Input: part model. Units: mm. Frame: model coordinates. Coordinates: 2 decimals unless noted, no trailing zeros. Write each loop counter-clockwise with the first axis right and the second up, starting at its lowest first coordinate (ties: lowest second). Pieces come first, ordered by that corner, then holes. Notation, with made-up numbers: (1.5, -36.5) - (24.5, -36.5) arc R28 ccw to (24.5, -13.5) - close; hole circle Ø9 at (-3.5, 89.25). An arc over 180 degrees is marked (long way). One line per question, with ' | ' between items. Start each with the question number.
1) Section query C-C on z = -72.5. Return loops of the section in (x, y).
2) Section query D-D on y = 1.4. Give the number of separate pieces and of enclosed holes in the cut face, and give its area (3 significant figures).
3) Line query: line 1 (X direction, y = 1.5, z = -33.5); line 2 (X direction, y = 0.4, z = 25); line 3 (X direction, y = 1.3, z = 7). Output: solid intervals per line, ascending.
4) Section query A-A on z = -9. Return loops of the section in (x, y).
5) First-contact query: P1, Ø1.5, axis at x = 33, z = 14.5, coming from the -Y side. Flat tip, straight axial feed; report the tip coordinate or a pass-through.
6) Section query B-B on x = 53. Return loops of the section in (y, z), and give its area (3 significant figures).
```python
from build123d import *

# Parameters (mm, degrees)
SKETCH3_W           = 200
SKETCH3_H           = 200
BOSS_EXTRUDE1_DEPTH = 3
SKETCH4_R           = 1.5
SKETCH4_R_2         = 23.5
SKETCH4_R_3         = 60
SKETCH4_W           = 30
SKETCH4_H           = 70
CUT_EXTRUDE1_DEPTH  = 5
FILLET1_R           = 5
FILLET2_R           = 2
CUT_EXTRUDE2_START  = -1
CUT_EXTRUDE2_DEPTH  = 1


with BuildPart() as part:
    # Sketch3 → Boss-Extrude1 (new body)
    with BuildSketch(Plane(origin=(0, 0, 0), x_dir=(1, 0, 0), z_dir=(0, 1, 0))):
        Rectangle(SKETCH3_W, SKETCH3_H)
    extrude(amount=BOSS_EXTRUDE1_DEPTH)

    # Sketch4 → Cut-Extrude1 (cut)
    with BuildSketch(Plane(origin=(0, 3, 0), x_dir=(1, 0, 0), z_dir=(0, 1, 0))):
        with Locations(Location((92, 92, 0), (0, 0, 270))):
            Circle(SKETCH4_R)
        with Locations(Location((92, -92, 0), (0, 0, 270))):
            Circle(SKETCH4_R)
        with Locations(Location((-92, -92, 0), (0, 0, 270))):
            Circle(SKETCH4_R)
        with Locations(Location((-92, 92, 0), (0, 0, 270))):
            Circle(SKETCH4_R)
        with Locations(Location((92, -25, 0), (0, 0, 270))):
            Circle(SKETCH4_R)
        with Locations(Location((93.5, -65, 0), (0, 0, 270))):
            Circle(SKETCH4_R)
        with Locations(Location((17, -93, 0), (0, 0, 270))):
            Circle(SKETCH4_R)
        with Locations(Location((29, -73, 0), (0, 0, 270))):
            Circle(SKETCH4_R)
        with Locations(Location((75, 92, 0), (0, 0, 270))):
            Circle(SKETCH4_R)
        with Locations(Location((29, -27, 0), (0, 0, 270))):
            Circle(SKETCH4_R)
        with Locations(Location((17, -7, 0), (0, 0, 270))):
            Circle(SKETCH4_R)
        with Locations(Location((-92, -25, 0), (0, 0, 270))):
            Circle(SKETCH4_R)
        with Locations(Location((-17, -93, 0), (0, 0, 270))):
            Circle(SKETCH4_R)
        with Locations(Location((-29, -73, 0), (0, 0, 270))):
            Circle(SKETCH4_R)
        with Locations(Location((-29, -27, 0), (0, 0, 270))):
            Circle(SKETCH4_R)
        with Locations(Location((-17, -7, 0), (0, 0, 270))):
            Circle(SKETCH4_R)
        with Locations(Location((65, -65, 0), (0, 0, 270))):
            Circle(SKETCH4_R_2)
        with Locations(Location((65, -93.5, 0), (0, 0, 270))):
            Circle(SKETCH4_R)
        with Locations(Location((36.5, -65, 0), (0, 0, 270))):
            Circle(SKETCH4_R)
        with Locations(Location((65, -36.5, 0), (0, 0, 270))):
            Circle(SKETCH4_R)
        with Locations(Location((57, 16.85, 0), (0, 0, 270))):
            Circle(SKETCH4_R)
        with Locations(Location((57, 33.15, 0), (0, 0, 270))):
            Circle(SKETCH4_R)
        with Locations(Location((43, 16.85, 0), (0, 0, 270))):
            Circle(SKETCH4_R)
        with Locations(Location((43, 33.15, 0), (0, 0, 270))):
            Circle(SKETCH4_R)
        with Locations((0, 100)):
            Circle(SKETCH4_R_3)
        with Locations(Location((-75, 92, 0), (0, 0, 270))):
            Circle(SKETCH4_R)
        with Locations(Location((0, 0, 0), (0, 0, 270))):
            Circle(SKETCH4_R)
        with Locations((85, 25)):
            Rectangle(SKETCH4_W, SKETCH4_H)
    cut_extrude1 = extrude(amount=-CUT_EXTRUDE1_DEPTH, mode=Mode.SUBTRACT)

    # Mirror1: Cut-Extrude1 across plane
    add(cut_extrude1.mirror(Plane.ZY), mode=Mode.SUBTRACT)

    # Fillet1
    fillet1_edges = [part.edges().sort_by_distance(p)[0] for p in [
        (-100, 1.5, 10),
        (-100, 1.5, -60),
        (-100, 1.5, -100),
        (100, 1.5, -100),
        (100, 1.5, 100),
        (-100, 1.5, 100),
        (60, 1.5, -100),
        (-60, 1.5, -100),
        (100, 1.5, -60),
        (100, 1.5, 10),
    ]]
    fillet(fillet1_edges, radius=FILLET1_R)

    # Fillet2
    fillet2_edges = [part.edges().sort_by_distance(p)[0] for p in [
        (-70, 1.5, -60),
        (-70, 1.5, 10),
        (70, 1.5, 10),
        (70, 1.5, -60),
    ]]
    fillet(fillet2_edges, radius=FILLET2_R)

    # Sketch5 → Cut-Extrude2 (cut)
    with BuildSketch(Plane(origin=(0, 3, 0), x_dir=(1, 0, 0), z_dir=(0, 1, 0)).offset(CUT_EXTRUDE2_START)):
        with BuildLine():
            Line((-95, -100), (95, -100))
            ThreePointArc((95, -100), (98.535533906, -98.535533906), (100, -95))
            Line((100, -95), (100, -15))
            ThreePointArc((100, -15), (98.535533906, -11.464466094), (95, -10))
            Line((95, -10), (72, -10))
            ThreePointArc((72, -10), (70.585786438, -9.414213562), (70, -8))
            Line((70, -8), (70, 58))
            ThreePointArc((70, 58), (70.585786438, 59.414213562), (72, 60))
            Line((72, 60), (95, 60))
            ThreePointArc((95, 60), (98.535533906, 61.464466094), (100, 65))
            Line((100, 65), (100, 95))
            ThreePointArc((100, 95), (98.535533906, 98.535533906), (95, 100))
            Line((95, 100), (64.807406984, 100))
            ThreePointArc((64.807406984, 100), (61.410575882, 98.668996929), (59.822221831, 95.384615385))
            ThreePointArc((59.822221831, 95.384615385), (0, 40), (-59.822221831, 95.384615385))
            ThreePointArc((-59.822221831, 95.384615385), (-61.410575882, 98.668996929), (-64.807406984, 100))
            Line((-64.807406984, 100), (-95, 100))
            ThreePointArc((-95, 100), (-98.535533906, 98.535533906), (-100, 95))
            Line((-100, 95), (-100, 65))
            ThreePointArc((-100, 65), (-98.535533906, 61.464466094), (-95, 60))
            Line((-95, 60), (-72, 60))
            ThreePointArc((-72, 60), (-70.585786438, 59.414213562), (-70, 58))
            Line((-70, 58), (-70, -8))
            ThreePointArc((-70, -8), (-70.585786438, -9.414213562), (-72, -10))
            Line((-72, -10), (-95, -10))
            ThreePointArc((-95, -10), (-98.535533906, -11.464466094), (-100, -15))
            Line((-100, -15), (-100, -95))
            ThreePointArc((-100, -95), (-98.535533906, -98.535533906), (-95, -100))
        make_face()
        with BuildLine():
            Line((-97, 95), (-97, 65))
            ThreePointArc((-97, 65), (-96.414213562, 63.585786438), (-95, 63))
            Line((-95, 63), (-72, 63))
            ThreePointArc((-72, 63), (-68.464466094, 61.535533906), (-67, 58))
            Line((-67, 58), (-67, -8))
            ThreePointArc((-67, -8), (-68.464466094, -11.535533906), (-72, -13))
            Line((-72, -13), (-95, -13))
            ThreePointArc((-95, -13), (-96.414213562, -13.585786438), (-97, -15))
            Line((-97, -15), (-97, -95))
            ThreePointArc((-97, -95), (-96.414213562, -96.414213562), (-95, -97))
            Line((-95, -97), (95, -97))
            ThreePointArc((95, -97), (96.414213562, -96.414213562), (97, -95))
            Line((97, -95), (97, -15))
            ThreePointArc((97, -15), (96.414213562, -13.585786438), (95, -13))
            Line((95, -13), (72, -13))
            ThreePointArc((72, -13), (68.464466094, -11.535533906), (67, -8))
            Line((67, -8), (67, 58))
            ThreePointArc((67, 58), (68.464466094, 61.535533906), (72, 63))
            Line((72, 63), (95, 63))
            ThreePointArc((95, 63), (96.414213562, 63.585786438), (97, 65))
            Line((97, 65), (97, 95))
            ThreePointArc((97, 95), (96.414213562, 96.414213562), (95, 97))
            Line((95, 97), (64.807406984, 97))
            ThreePointArc((64.807406984, 97), (63.448674543, 96.467598771), (62.813332923, 95.153846154))
            ThreePointArc((62.813332923, 95.153846154), (0, 37), (-62.813332923, 95.153846154))
            ThreePointArc((-62.813332923, 95.153846154), (-63.448674543, 96.467598771), (-64.807406984, 97))
            Line((-64.807406984, 97), (-95, 97))
            ThreePointArc((-95, 97), (-96.414213562, 96.414213562), (-97, 95))
        make_face(mode=Mode.SUBTRACT)
    extrude(amount=CUT_EXTRUDE2_DEPTH, mode=Mode.SUBTRACT)


solid = part.part
```
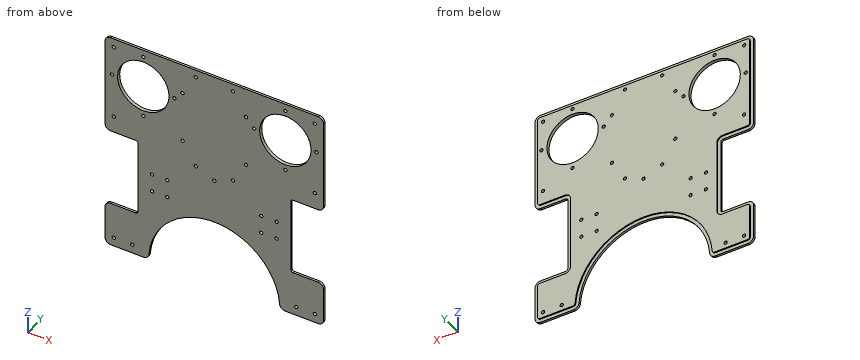
Answer key:
1) outline: (-100, 0) - (-53.33, 0) - (-53.33, 2) - (-56.68, 2) - (-56.68, 3) - (-97, 3) - (-97, 2) - (-100, 2) - close; (53.33, 0) - (100, 0) - (100, 2) - (97, 2) - (97, 3) - (56.68, 3) - (56.68, 2) - (53.33, 2) - close
2) separate pieces: 1 | enclosed holes: 35 | area: 26,400 mm²
3) line 1: -70 to -58.46, -55.54 to -44.46, -41.54 to 41.54, 44.46 to 55.54, 58.46 to 70 | line 2: -100 to -93.5, -90.5 to 90.5, 93.5 to 100 | line 3: -70 to -18.5, -15.5 to 15.5, 18.5 to 70
4) outline: (-70, 0) - (70, 0) - (70, 2) - (67, 2) - (67, 3) - (-67, 3) - (-67, 2) - (-70, 2) - close
5) P1: y = 0
6) outline: (0, -71.88) - (2, -71.88) - (2, -65.94) - (3, -65.94) - (3, 44.79) - (0, 44.79) - close; (0, 85.21) - (3, 85.21) - (3, 97) - (2, 97) - (2, 100) - (0, 100) - close | area: 385 mm²
